The model under review builds one solid part; all positions refer to its coordinate system, in mm. Face numbers are marked on the shaded views. A direction names the side the tool comes from. Coordinates: 2 decimals unless noted, no trailing zeros. Write each loop counter-clockwise with the first axis right and the second up, starting at its lowest first coordinate (ties: lowest second). Pieces come first, ordered by that corner, then holes.
1) Add section C-C, the plane y = 15.5. State the section outline as (x, z) points, then the cut area to 3 significant figures.
2) Add section A-A, the plane x = 0. State the section outline as (y, z) points.
3) Mouldability with a two-part tool opening along Y and no side actions: class the marked faces 3, 4, 5 and 6 as released by +Y, released by -Y, zero draft, split by the parting line, or undercut.
4) For line 1 (X direction, y = 17.5, z = 14.25); line 2 (Y direction, x = 0, z = 12.5); line 3 (Y direction, x = 8, z = 18.75), list the stretches that pass through material, from the lowest coordinate up.
5) Machinability: for the marked faces 1 and 2, which of the approach directions +Z, -Z, +X, -X, +Y, -Y give a long, thin tool a straight path to every point of the face, cutting with its end or side? Answer none if there is none.
6) For P1, Ø1, axis at x = 77, z = 16.5, coming from the -Y side; P2, Ø1, axis at y = 8.5, z = 5, coming from the -X side; P3, Ø8, axis at x = -28, z = 4, coming from the +Y side, all flat-tipped, find the tip position at first contact; note any pin that passes through.
7) Add section B-B, the plane y = 0. State the section outline as (x, z) points, then the cut area to 3 significant figures.
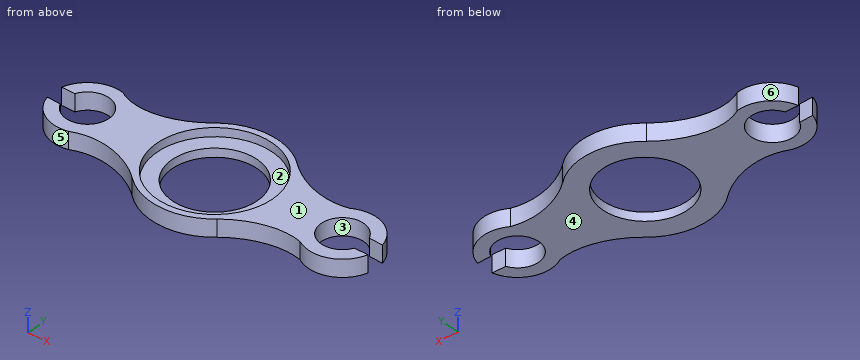
from build123d import *

# Parameters (mm, degrees)
SKETCH1_R            = 67.8
BOSS_EXTRUDE11_DEPTH = 20
SKETCH1_14_R         = 67.8
SKETCH1_14_R_2       = 50
BOSS_EXTRUDE12_DEPTH = 10


with BuildPart() as part:
    # Sketch1 → Boss-Extrude11 (new body)
    with BuildSketch(Plane.XY):
        with BuildLine():
            ThreePointArc((-142.34841847, 39.793144177), (-171.751198945, 34.54231297), (-189.319803444, 10.387833799))
            Line((-189.319803444, 10.387833799), (-173.788179779, 10.509033195))
            ThreePointArc((-173.788179779, 10.509033195), (-125.263414989, 1.225516677), (-173.304176626, -10.303650604))
            Line((-173.304176626, -10.303650604), (-189.176390414, -9.665625813))
            ThreePointArc((-189.176390414, -9.665625813), (-170.488139493, -34.024955882), (-140.039484135, -37.962857708))
            add(Edge.make_bspline(
                [(-140.039484135, -37.962857708), (-110.680407711, -24.08950974), (-74.045313114, -35.434332747), (-50.174260477, -55.547410213)],
                knots=[0.026307931, 0.026307931, 0.026307931, 0.026307931, 0.97051711, 0.97051711, 0.97051711, 0.97051711], degree=3))
            ThreePointArc((-50.174260477, -55.547410213), (0, -74.85299724), (50.174260477, -55.547410213))
            add(Edge.make_bspline(
                [(50.174260477, -55.547410213), (71.323341509, -37.727789453), (102.491508086, -26.790776239), (129.742096758, -34.176303824)],
                knots=[0.133974342, 0.133974342, 0.133974342, 0.133974342, 0.97051711, 0.97051711, 0.97051711, 0.97051711], degree=3))
            ThreePointArc((129.742096758, -34.176303824), (165.435107978, -37.117723558), (189.176390414, -10.303650604))
            Line((189.176390414, -10.303650604), (173.304176626, -10.303650604))
            ThreePointArc((173.304176626, -10.303650604), (125.526231498, 0), (173.304176626, 10.303650604))
            Line((173.304176626, 10.303650604), (189.319803444, 9.749809007))
            ThreePointArc((189.319803444, 9.749809007), (165.700168673, 37.010155777), (129.742096758, 34.176303824))
            add(Edge.make_bspline(
                [(129.742096758, 34.176303824), (102.491508086, 26.790776239), (71.323341509, 37.727789453), (50.174260477, 55.547410213)],
                knots=[0.133974342, 0.133974342, 0.133974342, 0.133974342, 0.97051711, 0.97051711, 0.97051711, 0.97051711], degree=3))
            ThreePointArc((50.174260477, 55.547410213), (0.430867535, 74.851757154), (-49.531464066, 56.121344098))
            add(Edge.make_bspline(
                [(-49.531464066, 56.121344098), (-73.874099433, 35.650364126), (-112.8184932, 22.464713449), (-142.34841847, 39.793144177)],
                knots=[1, 1, 1, 1, 1.97887484, 1.97887484, 1.97887484, 1.97887484], degree=3))
        make_face()
        Circle(SKETCH1_R, mode=Mode.SUBTRACT)
    extrude(amount=BOSS_EXTRUDE11_DEPTH)

    # Sketch1_14 → Boss-Extrude12 (add)
    with BuildSketch(Plane.XY):
        Circle(SKETCH1_14_R)
        Circle(SKETCH1_14_R_2, mode=Mode.SUBTRACT)
    extrude(amount=BOSS_EXTRUDE12_DEPTH)


solid = part.part
Geometry results:
1. outline: (-187.66, 0) - (-170.96, 0) - (-170.96, 20) - (-187.66, 20) - close; (-130.09, 0) - (-47.54, 0) - (-47.54, 10) - (-66, 10) - (-66, 20) - (-130.09, 20) - close; (47.54, 0) - (130.91, 0) - (130.91, 20) - (66, 20) - (66, 10) - (47.54, 10) - close; (170.14, 0) - (187.4, 0) - (187.4, 20) - (170.14, 20) - close
1. area: 3,630 mm2
2. outline: (-74.85, 0) - (-50, 0) - (-50, 10) - (-67.8, 10) - (-67.8, 20) - (-74.85, 20) - close; (50, 0) - (74.85, 0) - (74.85, 20) - (67.8, 20) - (67.8, 10) - (50, 10) - close
3. face 3: undercut
3. face 4: zero draft
3. face 5: released by -Y
3. face 6: released by +Y
4. line 1: x = -186.8 to -169.35, -131.71 to -65.5, 65.5 to 132.67, 168.38 to 186.49
4. line 2: y = -74.85 to -67.8, 67.8 to 74.85
4. line 3: y = -74.42 to -67.33, 67.33 to 74.42
5. face 1: +Z, +X, -X, +Y, -Y
5. face 2: +Z
6. P1: stops at y = -39.41
6. P2: stops at x = -126.68
6. P3: stops at y = 70.9
7. outline: (-125.26, 0) - (-50, 0) - (-50, 10) - (-67.8, 10) - (-67.8, 20) - (-125.26, 20) - close; (50, 0) - (125.53, 0) - (125.53, 20) - (67.8, 20) - (67.8, 10) - (50, 10) - close
7. area: 2,660 mm2
